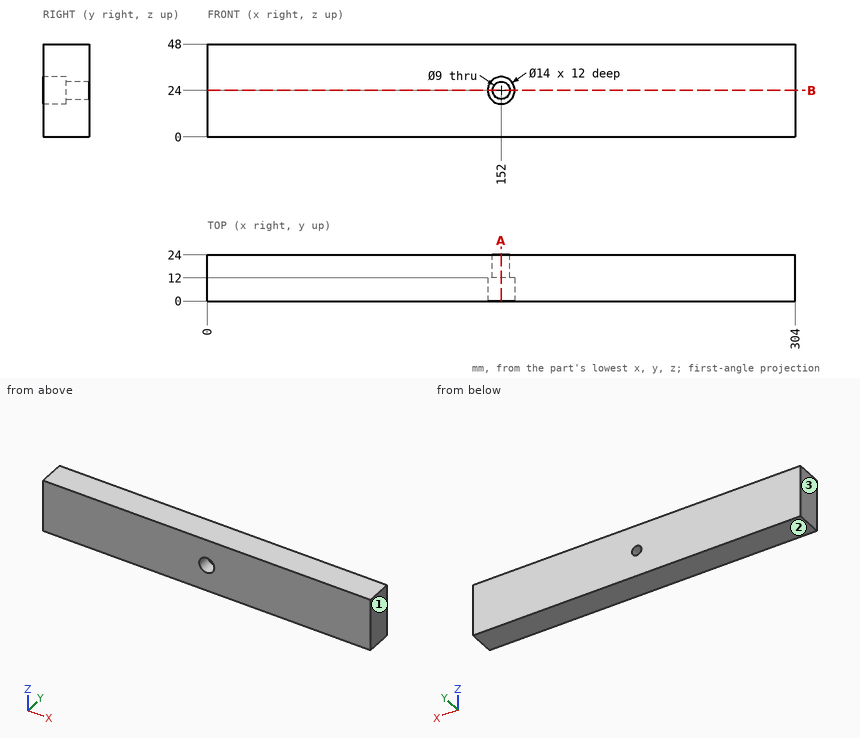
Source: three-view drawing plus pictorial views. Frame: mm from the lowest corner of the part. Give positions to 0.01 mm unless a question says otherwise; leave off trailing zeros. Write each loop counter-clockwise with the first axis right and the second up, starting at its lowest first coordinate (ties: lowest second). Pieces come first, ordered by that corner, then holes. Notation, with made-up numbers: (32, 48) -> (57, 48) arc R24 cw to (57, 74) -> close; hole circle Ø4 at (-12.5, -23.5). An arc over 180 degrees is marked (long way). Write item = value, one per line.
Q1. First-contact query: pin 1 (7 mm diameter, centred on x = 153.5, z = 23.5, fed in from -Y). Flat tip, straight axial feed; report the tip coordinate or a pass-through.
Here are the results:
pin_1 = 12
Q2. Line query: line 1 (X direction, y = 20.5, z = 24); line 2 (X direction, y = 7, z = 27). Output: solid intervals per line, ascending. Write a range as from..to.
Here are the results:
line_1 = 0..147.5, 156.5..304
line_2 = 0..145.68, 158.32..304
Q3. Mould query, pull axis X, two halves, no side actions, for the marked faces 1, 2 and 3. Classes: +X half, -X half, draft (parallel to the pull), parting line (faces both ways), or undercut.
Here are the results:
face_1 = +X half
face_2 = draft
face_3 = -X half
Q4. Cut plane A-A on x = 152. Return loops of the section in (y, z), then the cut area to 3 significant figures.
Here are the results:
outline = (0, 0) -> (24, 0) -> (24, 19.5) -> (12, 19.5) -> (12, 17) -> (0, 17) -> close; (0, 31) -> (12, 31) -> (12, 28.5) -> (24, 28.5) -> (24, 48) -> (0, 48) -> close
area = 876 mm²
Q5. Cut plane B-B on z = 24. Return loops of the section in (x, y), then the cut area to 3 significant figures.
Here are the results:
outline = (0, 0) -> (145, 0) -> (145, 12) -> (147.5, 12) -> (147.5, 24) -> (0, 24) -> close; (156.5, 12) -> (159, 12) -> (159, 0) -> (304, 0) -> (304, 24) -> (156.5, 24) -> close
area = 7,020 mm²
